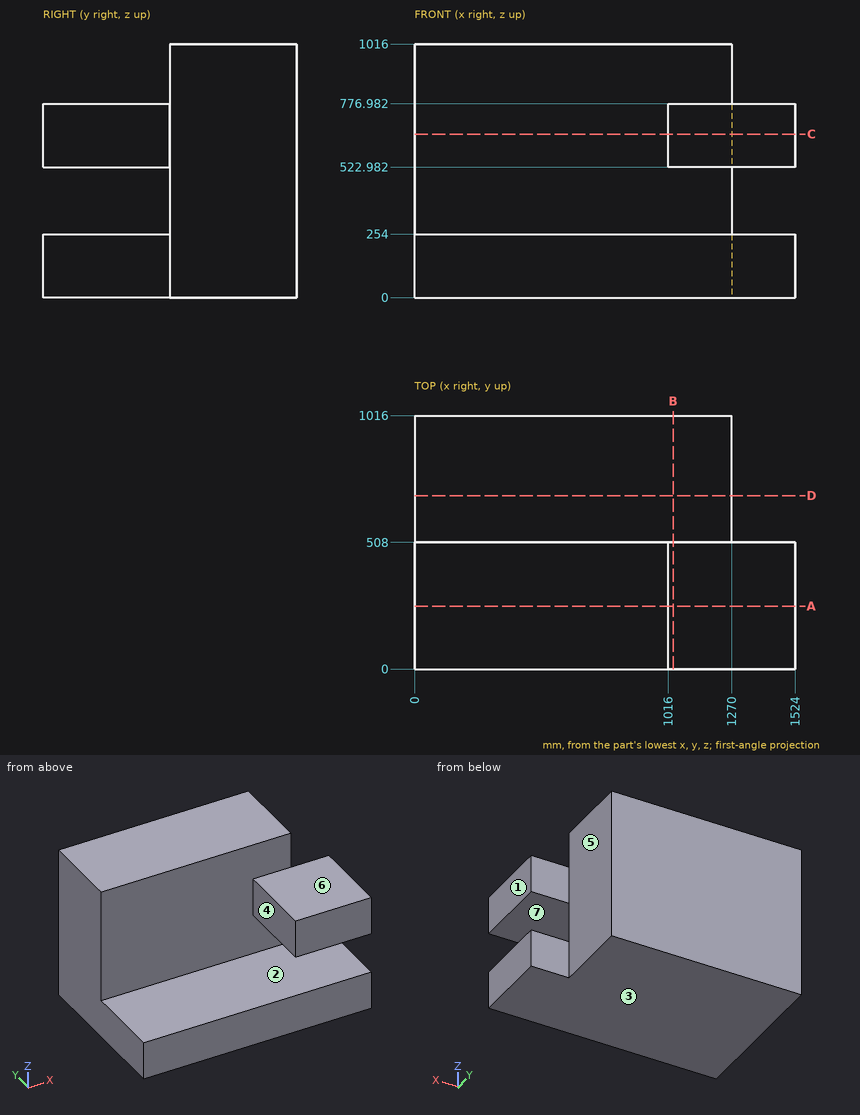
Geometry check sheet. Reference: drawing and pictorial views, mm from the part's lowest x, y, z. A direction names the side the tool comes from. Give positions to 0.01 mm unless a question says otherwise; leave off trailing zeros. Write each loop counter-clockwise with the first axis right and the second up, starting at its lowest first coordinate (ties: lowest second). Pieces come first, ordered by that corner, then holes. Notation, with made-up numbers: (-34, 19.25) - (-13, 19.25) arc R26 cw to (-13, 44.25) - close; hole circle Ø9 at (45.25, 0). An arc over 180 degrees is marked (long way). Use a Markdown table: item, result.
Q1. Section check C-C, the plane z = 654.5. Enter the section's corners in (x, y).
Computed:
| item | result |
|---|---|
| outline | (0, 508) - (1016, 508) - (1016, 0) - (1524, 0) - (1524, 508) - (1270, 508) - (1270, 1016) - (0, 1016) - close |
Q2. Section check D-D, the plane y = 695.5. Enter the section's corners in (x, z).
Computed:
| item | result |
|---|---|
| outline | (0, 0) - (1270, 0) - (1270, 1016) - (0, 1016) - close |
Q3. Thickness scan on L1, parallel to X at y = 167, z = 527; L2, parallel to Z at x = 607, y = 85; L3, parallel to Z at x = 1104.5, y = 111.5. Record the ranges inside material, lowest first. Write a range as [from, to].
Computed:
| item | result |
|---|---|
| L1 | x = [1016, 1524] |
| L2 | z = [0, 254] |
| L3 | z = [0, 254], [522.98, 776.98] |
Q4. Section check A-A, the plane y = 252.5. Enter the section's corners in (x, z).
Computed:
| item | result |
|---|---|
| outline | (0, 0) - (1524, 0) - (1524, 254) - (0, 254) - close; (1016, 522.98) - (1524, 522.98) - (1524, 776.98) - (1016, 776.98) - close |
Q5. Set-up check for the marked faces 4, 5, 6 and 7: record each of +Z, -Z, +X, -X, +Y, -Y from which the full face is reachable in a straight line by a thin tool's end or side.
Computed:
| item | result |
|---|---|
| face 4 | +Z, -X, -Y |
| face 5 | +Z, -Z, +X, +Y |
| face 6 | +Z, +X, -X, -Y |
| face 7 | +X, -X, -Y |
Q6. Section check B-B, the plane x = 1036. Enter the section's corners in (y, z), then the cut area to 3 significant figures.
Computed:
| item | result |
|---|---|
| outline | (0, 0) - (1016, 0) - (1016, 1016) - (508, 1016) - (508, 776.98) - (0, 776.98) - (0, 522.98) - (508, 522.98) - (508, 254) - (0, 254) - close |
| area | 774,000 mm² |
Q7. Draft check along Z on the marked faces 1, 2 and 3. Enter one of: pulls with the +Z half, pulls with the -Z half, needs draft (parallel to the pull), parting line crosses it, or undercut.
Computed:
| item | result |
|---|---|
| face 1 | needs draft |
| face 2 | undercut |
| face 3 | pulls with the -Z half |
